Here's the drawing with two shaded views (mm, measured from the low corner). I have some questions. A direction names the side the tool comes from. Coordinates: 2 decimals unless noted, no trailing zeros. Loops run counter-clockwise (first coordinate to the right, second up) from the corner with the lowest first, then second, coordinate; pieces in that order, holes last. Notation, with made-up numbers: (68.25, 13) -> (90.25, 13) arc R17 ccw to (90.25, 24) -> close; hole circle Ø8 at (42.25, 51.5). An arc over 180 degrees is marked (long way). Answer as a JSON object with one key per item and string values. Group by question number.
Q1. Thinking about a two-plate mould opening in X: for the marked faces 1, 2 and 3, which applies, released by +X, released by -X, zero draft, split by the parting line, or undercut?
Q2. I need wall thicknesses on line 1 (Y direction, x = 40, z = 3.15); line 2 (X direction, y = 14, z = 13.25); line 3 (Y direction, x = 10, z = 8.75). Which ranges of each line are inside material? Lowest first, please.
Q3. On a 3-axis mill with a long thin cutter (end or side, diameter ignored), from which of +Z, -Z, +X, -X, +Y, -Y can I reach the whole of each face in a straight line? I mean the marked faces 4 and 5. Say none if no direction works.
Q4. I want a section at B-B on x = 10. Write out the boundary of the cut face in (y, z).
Q5. I want a section at C-C on z = 2. Write out the boundary of the cut face in (x, y), then the cut area to 3 significant figures.
Q6. I want a section at A-A on z = 12.5. Write out the boundary of the cut face in (x, y), then the cut area to 3 significant figures.
Q7. I want a section at D-D on x = 40. Write out the boundary of the cut face in (y, z).
Q8. I'm going to push a flat-ended pin straight in: pin 1 (5 mm diameter, centred on x = 40, y = 10, fed in from +Z). Where does the tip first touch, or does it pass through?
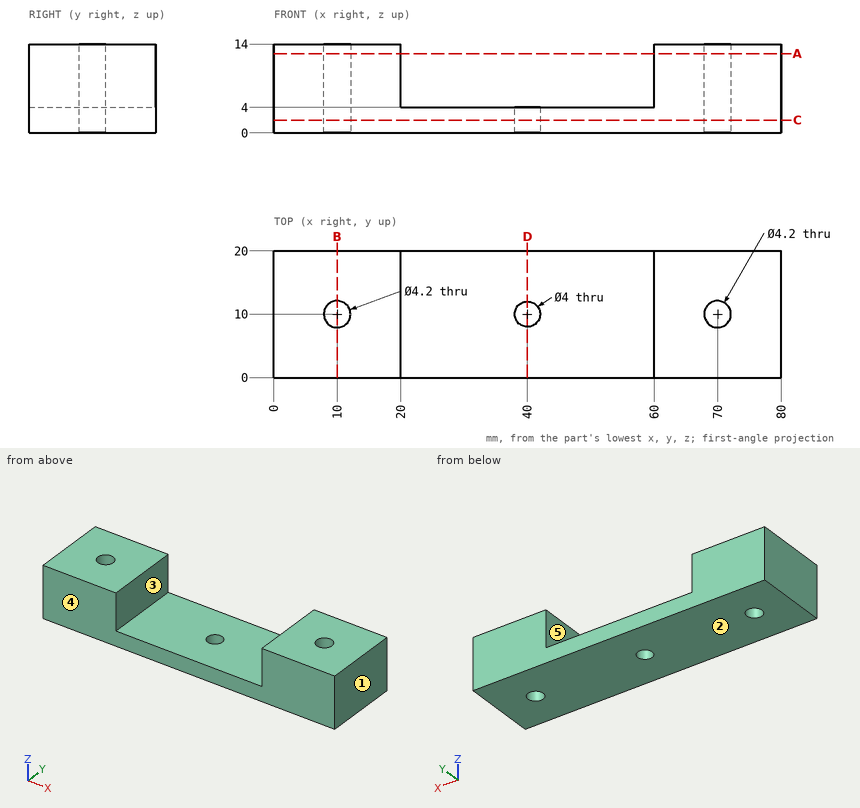
Result set:
{
 "1": {"face 1": "released by +X", "face 2": "zero draft", "face 3": "undercut"},
 "2": {"line 1": "y = 0 to 8, 12 to 20", "line 2": "x = 0 to 20, 60 to 80", "line 3": "y = 0 to 7.9, 12.1 to 20"},
 "3": {"face 4": "+Z, -Z, +X, -X, -Y", "face 5": "+Z, +Y, -Y"},
 "4": {"outline": "(0, 0) -> (7.9, 0) -> (7.9, 14) -> (0, 14) -> close; (12.1, 0) -> (20, 0) -> (20, 14) -> (12.1, 14) -> close"},
 "5": {"outline": "(0, 0) -> (80, 0) -> (80, 20) -> (0, 20) -> close; hole circle Ø4.2 at (10, 10); hole circle Ø4 at (40, 10); hole circle Ø4.2 at (70, 10)", "area": "1,560 mm²"},
 "6": {"outline": "(0, 0) -> (20, 0) -> (20, 20) -> (0, 20) -> close; (60, 0) -> (80, 0) -> (80, 20) -> (60, 20) -> close; hole circle Ø4.2 at (10, 10); hole circle Ø4.2 at (70, 10)", "area": "772 mm²"},
 "7": {"outline": "(0, 0) -> (8, 0) -> (8, 4) -> (0, 4) -> close; (12, 0) -> (20, 0) -> (20, 4) -> (12, 4) -> close"},
 "8": {"pin 1": "stops at z = 4"}
}
